```python
from build123d import *

# Parameters (mm, degrees)
SKETCH_1_W      = 130
SKETCH_1_H      = 17
SKETCH_1_R      = 3.5
SKETCH_1_R_2    = 1.15
EXTRUDE_1_DEPTH = 3
FILLET_1_R      = 3


with BuildPart() as part:
    # 草图1 → 凸台-拉伸1 (new body)
    with BuildSketch(Plane.XY):
        Rectangle(SKETCH_1_W, SKETCH_1_H)
        with Locations((-57, 0)):
            Circle(SKETCH_1_R, mode=Mode.SUBTRACT)
        with Locations((-45, 5)):
            Circle(SKETCH_1_R_2, mode=Mode.SUBTRACT)
        with Locations((-45, -5)):
            Circle(SKETCH_1_R_2, mode=Mode.SUBTRACT)
        with Locations((5, 6)):
            Circle(SKETCH_1_R_2, mode=Mode.SUBTRACT)
        with Locations((13, 6)):
            Circle(SKETCH_1_R_2, mode=Mode.SUBTRACT)
        with Locations((5, -6)):
            Circle(SKETCH_1_R_2, mode=Mode.SUBTRACT)
        with Locations((13, -6)):
            Circle(SKETCH_1_R_2, mode=Mode.SUBTRACT)
        with Locations((48, 6)):
            Circle(SKETCH_1_R_2, mode=Mode.SUBTRACT)
        with Locations((56, 6)):
            Circle(SKETCH_1_R_2, mode=Mode.SUBTRACT)
        with Locations((56, -6)):
            Circle(SKETCH_1_R_2, mode=Mode.SUBTRACT)
        with Locations((48, -6)):
            Circle(SKETCH_1_R_2, mode=Mode.SUBTRACT)
    extrude(amount=EXTRUDE_1_DEPTH)

    # 圆角1
    fillet_1_edges = [part.edges().sort_by_distance(p)[0] for p in [
        (65, -8.5, 1.5),
        (-65, -8.5, 1.5),
        (-65, 8.5, 1.5),
        (65, 8.5, 1.5),
    ]]
    fillet(fillet_1_edges, radius=FILLET_1_R)


solid = part.part
```
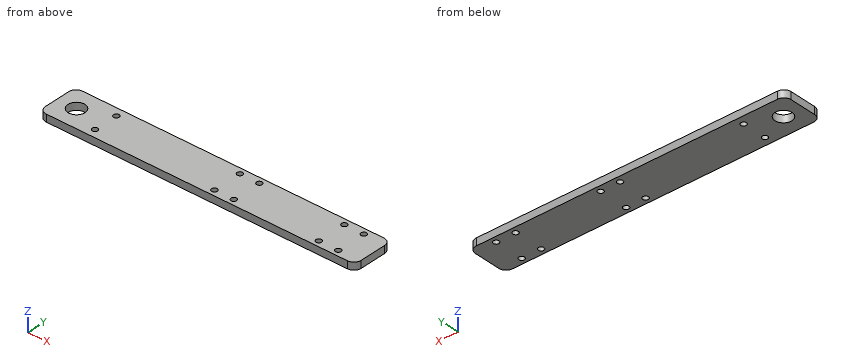
Model file for the job. Use its own axes, mm. Give positions to 0.01 mm unless a question says otherwise; leave off trailing zeros. Loops run counter-clockwise (first coordinate to the right, second up) from the corner with the lowest first, then second, coordinate; pieces in that order, holes last. Notation, with made-up numbers: (36.25, -15) - (55.25, -15) arc R29 ccw to (55.25, 20) - close; hole circle Ø10 at (41, -23). An arc over 180 degrees is marked (long way). One line per item, written item: value. Start each with the question number.
1. Slice it at A-A (x = 13). List the corners of the cut face in (y, z).
2. Slice it at B-B (z = 2.3). Give the number of separate pieces and of enclosed holes in the cut face, plus the area to 3 significant figures.
3. Pin check, flat tips, straight feed: pin 1 (2.5 mm diameter, centred on x = 48, y = 6, fed in from -Z); pin 2 (2 mm diameter, centred on x = 5, y = -6, fed in from +Z). Stop position of each tip, or through.
4. Probe L1, parallel to Y at x = 5, z = 1.6; L2, parallel to X at y = -5.75, z = 2.05; L3, parallel to X at y = 1, z = 1.65. List the from-to ranges inside material, lowest first. Write a range as from..to.
5. Slice it at C-C (x = -57). List the corners of the cut face in (y, z), plus the area to 3 significant figures.
6. Slice it at D-D (y = 1.5). List the corners of the cut face in (x, z).
Solution:
1. outline: (-8.5, 0) - (-7.15, 0) - (-7.15, 3) - (-8.5, 3) - close; (-4.85, 0) - (4.85, 0) - (4.85, 3) - (-4.85, 3) - close; (7.15, 0) - (8.5, 0) - (8.5, 3) - (7.15, 3) - close
2. separate pieces: 1
2. enclosed holes: 11
2. area: 2,120 mm^2
3. pin 1: stops at z = 0
3. pin 2: passes through
4. L1: y = -8.5..-7.15, -4.85..4.85, 7.15..8.5
4. L2: x = -64.99..-45.87, -44.13..3.88, 6.12..11.88, 14.12..46.88, 49.12..54.88, 57.12..64.99
4. L3: x = -65..-60.35, -53.65..65
5. outline: (-8.5, 0) - (-3.5, 0) - (-3.5, 3) - (-8.5, 3) - close; (3.5, 0) - (8.5, 0) - (8.5, 3) - (3.5, 3) - close
5. area: 30.0 mm^2
6. outline: (-65, 0) - (-60.16, 0) - (-60.16, 3) - (-65, 3) - close; (-53.84, 0) - (65, 0) - (65, 3) - (-53.84, 3) - close
